```python
from build123d import *

# Parameters (mm, degrees)
SKETCH1_W                                      = 306.05
SKETCH1_H                                      = 197.425
SKETCH1_R                                      = 10.775
BOSS_EXTRUDE1_DEPTH                            = 2.38125
SKETCH9_W                                      = 306.05
SKETCH9_H                                      = 2.38125
BOSS_EXTRUDE2_DEPTH                            = 3.175
SKETCH10_R                                     = 3.5
CUT_EXTRUDE1_DEPTH                             = 184.856965146
CSK_FOR_M3_FLAT_HEAD_MACHINE_SCREW1_AT_2_COUNT = 2
CSK_FOR_M3_FLAT_HEAD_MACHINE_SCREW1_AT_2_PITCH = 28.69
CSK_FOR_M3_FLAT_HEAD_MACHINE_SCREW1_AT_3_COUNT = 2
CSK_FOR_M3_FLAT_HEAD_MACHINE_SCREW1_AT_3_PITCH = 178.948509983
CSK_FOR_M3_FLAT_HEAD_MACHINE_SCREW1_AT_4_COUNT = 2
CSK_FOR_M3_FLAT_HEAD_MACHINE_SCREW1_AT_4_PITCH = 208.645558843
CSK_FOR_M3_FLAT_HEAD_MACHINE_SCREW1_AT_5_COUNT = 2
CSK_FOR_M3_FLAT_HEAD_MACHINE_SCREW1_AT_5_PITCH = 260.467597265
CSK_FOR_M3_FLAT_HEAD_MACHINE_SCREW1_AT_6_COUNT = 2
CSK_FOR_M3_FLAT_HEAD_MACHINE_SCREW1_AT_6_PITCH = 224.342
CSK_FOR_M3_FLAT_HEAD_MACHINE_SCREW1_AT_7_COUNT = 2
CSK_FOR_M3_FLAT_HEAD_MACHINE_SCREW1_AT_7_PITCH = 195.652
SKETCH13_R                                     = 6
CUT_EXTRUDE2_DEPTH                             = 184.856965146


with BuildPart() as part:
    # Sketch1 → Boss-Extrude1 (new body)
    # profile 1 of 5: a face of its own
    with BuildSketch(Plane.XY):
        Rectangle(SKETCH1_W, SKETCH1_H)
        with Locations((-142.25, -87.9375)):
            Circle(SKETCH1_R, mode=Mode.SUBTRACT)
        with Locations((-130.25, -64.9375)):
            Circle(SKETCH1_R, mode=Mode.SUBTRACT)
    # profile 2 of 5: a face of its own
    with BuildSketch(Plane.XY):
        with Locations((-130.25, -64.9375)):
            Circle(SKETCH1_R)
    # profile 3 of 5: a face of its own
    with BuildSketch(Plane.XY):
        with Locations((-142.25, -87.9375)):
            Circle(SKETCH1_R)
    # profile 4 of 5: a face of its own
    with BuildSketch(Plane.XY):
        with BuildLine():
            ThreePointArc((-142.25, -98.7125), (-149.869075567, -95.556575567), (-153.025, -87.9375))
            Line((-153.025, -87.9375), (-153.025, -98.7125))
            Line((-153.025, -98.7125), (-142.25, -98.7125))
        make_face()
    # profile 5 of 5: a face of its own
    with BuildSketch(Plane.XY):
        Rectangle(SKETCH1_W, SKETCH1_H)
    extrude(amount=BOSS_EXTRUDE1_DEPTH)

    # Sketch9 → Boss-Extrude2 (add)
    with BuildSketch(Plane(origin=(0, 98.7125, 0), x_dir=(1, 0, 0), z_dir=(0, 1, 0))):
        with Locations((0, -1.190625)):
            Rectangle(SKETCH9_W, SKETCH9_H)
    extrude(amount=BOSS_EXTRUDE2_DEPTH)

    # Sketch10 → Cut-Extrude1 (cut, through all)
    with BuildSketch(Plane(origin=(0, 0, 0), x_dir=(-1, 0, 0), z_dir=(0, 0, -1))):
        with Locations((-134.610000066, 92.3625)):
            Circle(SKETCH10_R)
        with Locations((-124.450000066, 92.3625)):
            Circle(SKETCH10_R)
        with Locations((-143.817500066, -87.5375001)):
            Circle(SKETCH10_R)
        with Locations((-133.657500066, -87.5375001)):
            Circle(SKETCH10_R)
    cut_extrude1 = extrude(amount=-CUT_EXTRUDE1_DEPTH, mode=Mode.SUBTRACT)

    # Mirror1: Cut-Extrude1 across plane
    add(cut_extrude1.mirror(Plane(origin=(0, 0, 0), x_dir=(0, 0, 1), z_dir=(1, 0, 0))), mode=Mode.SUBTRACT)

    # Sketch12 → CSK for M3 Flat Head Machine Screw1 (revolve, cut)
    with BuildSketch(Plane(origin=(111.94, -83.7125, 0), x_dir=(0, 1, 0), z_dir=(1, 0, 0))):
        Polygon((0, 0), (0, 2.38125), (1.7, 2.38125), (1.7, 1.45), (3.15, 0), align=None)
    csk_for_m3_flat_head_machine_screw1 = revolve(axis=Axis((111.94, -83.7125, -6.35), (0, 0, 1)), mode=Mode.SUBTRACT)

    # CSK for M3 Flat Head Machine Screw1 at 2: CSK for M3 Flat Head Machine Screw1 ×2
    with Locations(*[(-i * CSK_FOR_M3_FLAT_HEAD_MACHINE_SCREW1_AT_2_PITCH, 0, 0) for i in range(1, CSK_FOR_M3_FLAT_HEAD_MACHINE_SCREW1_AT_2_COUNT)]):
        add(csk_for_m3_flat_head_machine_screw1, mode=Mode.SUBTRACT)

    # CSK for M3 Flat Head Machine Screw1 at 3: CSK for M3 Flat Head Machine Screw1 ×2
    with Locations(*[Vector(-0.17848709666869053, 0.9839422525345589, 0) * (i * CSK_FOR_M3_FLAT_HEAD_MACHINE_SCREW1_AT_3_PITCH) for i in range(1, CSK_FOR_M3_FLAT_HEAD_MACHINE_SCREW1_AT_3_COUNT)]):
        add(csk_for_m3_flat_head_machine_screw1, mode=Mode.SUBTRACT)

    # CSK for M3 Flat Head Machine Screw1 at 4: CSK for M3 Flat Head Machine Screw1 ×2
    with Locations(*[Vector(-0.5365079449598512, 0.8438952689729675, 0) * (i * CSK_FOR_M3_FLAT_HEAD_MACHINE_SCREW1_AT_4_PITCH) for i in range(1, CSK_FOR_M3_FLAT_HEAD_MACHINE_SCREW1_AT_4_COUNT)]):
        add(csk_for_m3_flat_head_machine_screw1, mode=Mode.SUBTRACT)

    # CSK for M3 Flat Head Machine Screw1 at 5: CSK for M3 Flat Head Machine Screw1 ×2
    with Locations(*[Vector(-0.7369054808176358, 0.6759957931384847, 0) * (i * CSK_FOR_M3_FLAT_HEAD_MACHINE_SCREW1_AT_5_PITCH) for i in range(1, CSK_FOR_M3_FLAT_HEAD_MACHINE_SCREW1_AT_5_COUNT)]):
        add(csk_for_m3_flat_head_machine_screw1, mode=Mode.SUBTRACT)

    # CSK for M3 Flat Head Machine Screw1 at 6: CSK for M3 Flat Head Machine Screw1 ×2
    with Locations(*[(-i * CSK_FOR_M3_FLAT_HEAD_MACHINE_SCREW1_AT_6_PITCH, 0, 0) for i in range(1, CSK_FOR_M3_FLAT_HEAD_MACHINE_SCREW1_AT_6_COUNT)]):
        add(csk_for_m3_flat_head_machine_screw1, mode=Mode.SUBTRACT)

    # CSK for M3 Flat Head Machine Screw1 at 7: CSK for M3 Flat Head Machine Screw1 ×2
    with Locations(*[(-i * CSK_FOR_M3_FLAT_HEAD_MACHINE_SCREW1_AT_7_PITCH, 0, 0) for i in range(1, CSK_FOR_M3_FLAT_HEAD_MACHINE_SCREW1_AT_7_COUNT)]):
        add(csk_for_m3_flat_head_machine_screw1, mode=Mode.SUBTRACT)

    # Sketch13 → Cut-Extrude2 (cut, through all)
    with BuildSketch(Plane(origin=(0, 0, 0), x_dir=(-1, 0, 0), z_dir=(0, 0, -1))):
        with Locations((-97.75, -79.7125001)):
            Circle(SKETCH13_R)
        with Locations((97.75, -79.7125001)):
            Circle(SKETCH13_R)
    extrude(amount=-CUT_EXTRUDE2_DEPTH, mode=Mode.SUBTRACT)


solid = part.part
```
Part model, mm, in its own coordinate system. Coordinates: 2 decimals unless noted, no trailing zeros. Return JSON: item names as keys, results as strings. Group by question number.
Item 1: Pull direction X, two halves, no side cores. Call faces 1 (the face through (-2, 0, 2.381)), 2 (the face through (141.936, -84.586, 1.174)): pulls with the +X half, pulls with the -X half, needs draft (parallel to the pull), parting line crosses it, or undercut.
Item 2: Drill centre lines: probe 1 along Y at (x, z) = (134.61, 1); probe 2 along X at (y, z) = (-77.5, 0.5) (3 decimals); probe 3 along Y at (x, z) = (-130.5, 1.3). Where is each one in solid material? Low to high. Write a range as from..to.
Item 3: Pin check, flat tips, straight feed: pin 1 (15.5 mm diameter, centred on x = -97.75, y = -79.71, fed in from +Z); pin 2 (4.5 mm diameter, centred on x = 0, y = 92.36, fed in from -Z); pin 3 (5.5 mm diameter, centred on x = 80, y = 92.36, fed in from -Z). Stop position of each tip, or through.
Check values:
{
 "1": {"face 1": "needs draft", "face 2": "undercut"},
 "2": {"probe 1": "y = -98.71..-90.91, -84.17..88.86, 95.86..101.89", "probe 2": "x = -153.025..-103.327, -92.173..92.173, 103.327..153.025", "probe 3": "y = -98.71..-89.05, -86.03..101.89"},
 "3": {"pin 1": "stops at z = 2.38", "pin 2": "stops at z = 0.9", "pin 3": "stops at z = 0.4"}
}
